```python
from build123d import *

# Parameters (mm, degrees)
BOSS_EXTRU_1_DEPTH         = 200
R_P_TITION_LIN_AIRE1_COUNT = 15
R_P_TITION_LIN_AIRE1_PITCH = 13.31
ESQUISSE4_OUTSIDE_W        = 258.204
ESQUISSE4_OUTSIDE_H        = 258.554
ENL_V_MAT_EXTRU_2_DEPTH    = 150


with BuildPart() as part:
    # Esquisse1 → Boss.-Extru.1 (new body)
    with BuildSketch(Plane(origin=(0, 0, 0), x_dir=(1, 0, 0), z_dir=(0, 1, 0))):
        Polygon((0, 10), (6.615825808, 3), (6.615825808, 0), (0, 7), (-6.694174192, 0), (-6.694174192, 3), align=None)
    boss_extru_1 = extrude(amount=BOSS_EXTRU_1_DEPTH)

    # Répétition linéaire1: Boss.-Extru.1 ×15
    with Locations(*[(i * R_P_TITION_LIN_AIRE1_PITCH, 0, 0) for i in range(1, R_P_TITION_LIN_AIRE1_COUNT)]):
        add(boss_extru_1)

    # Esquisse4 outside → Enlèv. mat.-Extru.2 (cut)
    with BuildSketch(Plane.XY.offset(-10)):
        with Locations((93.131, 100)):
            Rectangle(ESQUISSE4_OUTSIDE_W, ESQUISSE4_OUTSIDE_H)
        Polygon((66.55, 25.147148524), (159.72, 108.218978148), (106.48, 167.930806122), (13.31, 84.858976498), align=None, mode=Mode.SUBTRACT)
    extrude(amount=ENL_V_MAT_EXTRU_2_DEPTH, mode=Mode.SUBTRACT)


solid = part.part
```
CAD build for the part. Positions are in the model's coordinates, mm. A direction names the side the tool comes from. Give positions to 0.01 mm unless a question says otherwise; leave off trailing zeros. Loops run counter-clockwise (first coordinate to the right, second up) from the corner with the lowest first, then second, coordinate; pieces in that order, holes last. Notation, with made-up numbers: (-13, -25.75) - (-1, -25.75) arc R18 cw to (-1, -18.75) - close; hole circle Ø6 at (73.25, 75.5). An arc over 180 degrees is marked (long way). Put each result on its own line as item: value.
Q1. Slice it at A-A (x = 75). Give the cut face in (y, z), plus the area to 3 significant figures.
Filled in:
outline: (32.68, -4.92) - (139.86, -4.92) - (139.86, -1.92) - (32.68, -1.92) - close
area: 322 mm²
Q2. Slice it at B-B (z = -5). Give the number of separate pieces and of enclosed holes in the cut face, plus the area to 3 significant figures.
Filled in:
separate pieces: 22
enclosed holes: 0
area: 4,280 mm²
Q3. Flat gauge pins, fed straight in: pin 1 (1.5 mm diameter, centred on x = 98, z = -2, fed in from +Y); pin 2 (6 mm diameter, centred on x = 130.5, z = -5, fed in from -Y); pin 3 (1 mm diameter, centred on y = 88, z = -5, fed in from +X); pin 4 (1.5 mm diameter, centred on x = 121, z = -2.5, fed in from -Y). Where does each tip first touch, or does it go through?
Filled in:
pin 1: stops at y = 161.04
pin 2: stops at y = 79.58
pin 3: stops at x = 137.6
pin 4: passes through
Q4. Slice it at C-C (x = 51.5). Give the cut face in (y, z), plus the area to 3 significant figures.
Filled in:
outline: (42.03, -8.18) - (118.91, -8.18) - (118.91, -5.18) - (42.03, -5.18) - close
area: 231 mm²
Q5. Mould opens along X. For faces 3 (the face through (18.13, 84.01, -1.9)), 4 (the face through (112.92, 66.49, -2.06)), 5 (the face through (96.43, 104.63, -6.55)) say: pulls with the +X half, pulls with the -X half, needs draft (parallel to the pull), parting line crosses it, or undercut.
Filled in:
face 3: pulls with the -X half
face 4: pulls with the +X half
face 5: undercut
Q6. Probe line 1 along X through (y, z) = (37.5, -5.25); line 2 along X through (y, z) = (128.5, -9.5); line 3 along X through (y, z) = (42, -2). List the from-to ranges inside material, lowest first.
Filled in:
line 1: x = 55.54 to 57.73, 62.01 to 64.88, 68.2 to 71.04, 75.32 to 78.19
line 2: x = 66.07 to 67.02, 79.38 to 80.33, 92.69 to 93.64, 106 to 106.95, 119.31 to 120.26, 132.62 to 133.57
line 3: x = 57.97 to 61.77, 71.28 to 75.08, 84.59 to 85.45
Q7. Tool access for faces 1 (the face through (43.284, 80.569, -3.451)), 2 (the face through (43.19, 80.57, -6.55)): list every direction of +Z, -Z, +X, -X, +Y, -Y with a clear straight run to the whole face (end or side of a thin tool).
Filled in:
face 1: +Z, +Y, -Y
face 2: -Z, +Y, -Y
